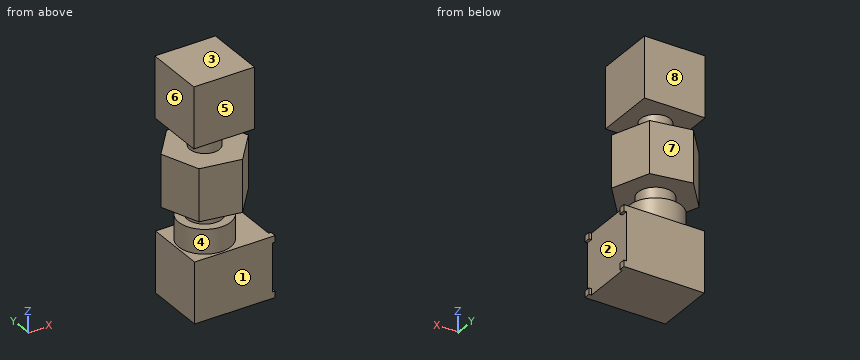
```python
from build123d import *

# Parameters (mm, degrees)
SKETCH1_W           = 9
SKETCH1_H           = 7
BOSS_EXTRUDE1_DEPTH = 7
SKETCH4_W           = 0.725
SKETCH4_H           = 0.725
BOSS_EXTRUDE3_DEPTH = 0.3
SKETCH_1_R          = 3
EXTRUDE_1_DEPTH     = 2.8
SKETCH_2_R          = 2
EXTRUDE_2_DEPTH     = 1.8
EXTRUDE_3_DEPTH     = 6
SKETCH_4_R          = 1.7
EXTRUDE_4_DEPTH     = 2.4
SKETCH_5_W          = 7
SKETCH_5_H          = 7
EXTRUDE_5_DEPTH     = 7


with BuildPart() as part:
    # Sketch1 → Boss-Extrude1 (new body)
    with BuildSketch(Plane(origin=(0, 0, 0), x_dir=(1, 0, 0), z_dir=(0, 1, 0))):
        Rectangle(SKETCH1_W, SKETCH1_H)
    extrude(amount=BOSS_EXTRUDE1_DEPTH)

    # Sketch4 → Boss-Extrude3 (add)
    with BuildSketch(Plane(origin=(4.5, 0, 0), x_dir=(0, 0, -1), z_dir=(1, 0, 0))):
        with Locations((-3.1375, 6.6375)):
            Rectangle(SKETCH4_W, SKETCH4_H)
        with Locations((3.1375, 6.6375)):
            Rectangle(SKETCH4_W, SKETCH4_H)
        with Locations((-3.1375, 0.3625)):
            Rectangle(SKETCH4_W, SKETCH4_H)
        with Locations((3.1375, 0.3625)):
            Rectangle(SKETCH4_W, SKETCH4_H)
    extrude(amount=BOSS_EXTRUDE3_DEPTH)

    # ｽｹｯﾁ1 → ﾎﾞｽ - 押し出し1 (add)
    with BuildSketch(Plane.XY.offset(3.5)):
        with Locations((-1.25, 3.25)):
            Circle(SKETCH_1_R)
    extrude(amount=EXTRUDE_1_DEPTH)

    # ｽｹｯﾁ2 → ﾎﾞｽ - 押し出し2 (add)
    with BuildSketch(Plane.XY.offset(6.3)):
        with Locations((-1.25, 3.25)):
            Circle(SKETCH_2_R)
    extrude(amount=EXTRUDE_2_DEPTH)

    # ｽｹｯﾁ3 → ﾎﾞｽ - 押し出し3 (add)
    with BuildSketch(Plane.XY.offset(8.1)):
        Polygon((1.697866371, 6.805758315), (-2.855443845, 7.580806321), (-5.803310216, 4.025048007), (-4.197866371, -0.305758315), (0.355443845, -1.080806321), (3.303310216, 2.474951993), align=None)
    extrude(amount=EXTRUDE_3_DEPTH)

    # ｽｹｯﾁ4 → ﾎﾞｽ - 押し出し4 (add)
    with BuildSketch(Plane.XY.offset(14.1)):
        with Locations((-1.25, 3.25)):
            Circle(SKETCH_4_R)
    extrude(amount=EXTRUDE_4_DEPTH)

    # ｽｹｯﾁ5 → ﾎﾞｽ - 押し出し5 (add)
    with BuildSketch(Plane.XY.offset(16.5)):
        with Locations((-1.25, 3.25)):
            Rectangle(SKETCH_5_W, SKETCH_5_H)
    extrude(amount=EXTRUDE_5_DEPTH)


solid = part.part
```
Verification items for the finished model (mm, model axes). Face numbers are marked on the shaded views. A direction names the side the tool comes from. Round coordinates to 2 decimals unless told otherwise and drop trailing zeros. Order: outer loops, then holes, each group sorted by start corner. A loop starts at its lowest first (then second) coordinate and runs counter-clockwise, first axis right, second up. Notation, with made-up numbers: (-10, 26.5) -> (39, 26.5) arc R13 ccw to (39, 48.5) -> close; hole circle Ø11 at (6, 87). An arc over 180 degrees is marked (long way). Put each result on its own line as item: value. Start each with the question number.
(1) Material ranges on line 1 along Z through (x, y) = (-1.5, 6); line 2 along Z through (x, y) = (1, 5.75); line 3 along Z through (x, y) = (2.5, 3.75), recorded low to high.
(2) Section check C-C (y = 3). Enter the section's corners in (x, z).
(3) Section check D-D (x = 3.75). Enter the section's corners in (y, z).
(4) Draft check along Z on the marked faces 1, 2 and 3. Enter one of: +Z half, -Z half, draft (parallel to the pull), parting line (faces both ways), or undercut.
(5) Section check A-A (y = 5.75). Enter the section's corners in (x, z), then the cut area to 3 significant figures.
(6) Depth check by flat-ended pin: pin 1 Ø3.5 at (x, z) = (-0.5, 21) entering from +Y; pin 2 Ø1.5 at (y, z) = (4.5, 2.5) entering from +X; pin 3 Ø5.5 at (x, z) = (0.5, 21.5) entering from -Y. Enter the tip coordinate at first touch or a pass-through.
(7) Tool access check on the marked faces 4, 5, 6, 7 and 8. Record the directions out of +Z, -Z, +X, -X, +Y, -Y that give a thin tool (end or side, any length) a straight path to the whole face; none if there is none.
(8) Section check B-B (z = 9). Enter the section's corners in (x, y), then the cut area to 3 significant figures.
Completed:
1. line 1: z = -3.5 to 6.3, 8.1 to 14.1, 16.5 to 23.5
1. line 2: z = -3.5 to 3.5, 8.1 to 14.1, 16.5 to 23.5
1. line 3: z = -3.5 to 3.5, 8.1 to 14.1
2. outline: (-5.42, 8.1) -> (-3.23, 8.1) -> (-3.23, 6.3) -> (-4.24, 6.3) -> (-4.24, 3.5) -> (-4.5, 3.5) -> (-4.5, -3.5) -> (4.5, -3.5) -> (4.5, 3.5) -> (1.74, 3.5) -> (1.74, 6.3) -> (0.73, 6.3) -> (0.73, 8.1) -> (3.11, 8.1) -> (3.11, 14.1) -> (0.43, 14.1) -> (0.43, 16.5) -> (2.25, 16.5) -> (2.25, 23.5) -> (-4.75, 23.5) -> (-4.75, 16.5) -> (-2.93, 16.5) -> (-2.93, 14.1) -> (-5.42, 14.1) -> close
3. outline: (0, -3.5) -> (7, -3.5) -> (7, 3.5) -> (0, 3.5) -> close
4. face 1: draft
4. face 2: undercut
4. face 3: +Z half
5. outline: (-4.75, 16.5) -> (2.25, 16.5) -> (2.25, 23.5) -> (-4.75, 23.5) -> close; (-4.5, -3.5) -> (4.5, -3.5) -> (4.5, 3.5) -> (0.41, 3.5) -> (0.41, 6.3) -> (-2.91, 6.3) -> (-2.91, 3.5) -> (-4.5, 3.5) -> close; (-4.37, 8.1) -> (2.09, 8.1) -> (2.09, 14.1) -> (-4.37, 14.1) -> close
5. area: 160 mm2
6. pin 1: stops at y = 6.75
6. pin 2: stops at x = 4.5
6. pin 3: stops at y = -0.25
7. face 4: none
7. face 5: +Z, +X, -X, -Y
7. face 6: +Z, -X, +Y, -Y
7. face 7: +Z, +X, +Y
7. face 8: +Z, +X, -X, +Y
8. outline: (-5.8, 4.03) -> (-4.2, -0.31) -> (0.36, -1.08) -> (3.3, 2.47) -> (1.7, 6.81) -> (-2.86, 7.58) -> close
8. area: 55.4 mm2
